For this review, take the finished solid that the model builds, in its own axes (mm). A direction names the side the tool comes from. Round coordinates to 2 decimals unless told otherwise and drop trailing zeros. Write each loop counter-clockwise with the first axis right and the second up, starting at its lowest first coordinate (ties: lowest second). Pieces come first, ordered by that corner, then holes. Notation, with made-up numbers: (-24, -26) -> (-12, -26) arc R20 ccw to (-12, -8) -> close; hole circle Ø5 at (-39.75, 74.25). An arc over 180 degrees is marked (long way). Write each question's results on one line, items separated by ' | '. Start each with the question number.
Item 1: To check wall thickness, follow line 1 along X through (y, z) = (107.5, 0) (3 decimals); line 2 along Y through (x, z) = (-3.5, -6); line 3 along X through (y, z) = (208, 4.75). State the ranges of each line that lie inside material, in increasing order.
Item 2: Add section B-B (y = 187). State the section outline as (x, z) points (3 decimals), plus the area to 3 significant figures.
Item 3: The part is to be moulded in two halves that separate along Z. For faces 1 (the cylindrical face through (3.86, 150.27, 5.04)), 2 (the cylindrical face through (1.93, 154.6, 2.52)), 3 (the flat face through (7, 304.8, 0)), say which applies: +Z half, -Z half, draft (parallel to the pull), parting line (faces both ways), or undercut.
Item 4: Add section A-A (x = 0). State the section outline as (y, z) points (3 decimals), plus the area to 3 significant figures.
Item 5: Clearance check with flat-ended pins moving along their axes: pin 1 (8 mm diameter, centred on x = 3, y = 146.5, fed in from -Z); pin 2 (2 mm diameter, centred on x = 5.5, y = 103.5, fed in from +Z); pin 3 (2 mm diameter, centred on x = 2, y = 65.5, fed in from +Z). State where each tip first meets the part, or that it passes through.
Item 6: Tool access review of faces 4 (the flat face through (7, 0, 0)), 5 (the flat face through (2, 309.8, -3)): name each direction out of +Z, -Z, +X, -X, +Y, -Y from which nothing blocks a thin tool from reaching the whole face with its end or side.
from build123d import *

# Parameters (mm, degrees)
SKETCH1_R            = 6.35
SKETCH1_R_2          = 3.175
BOSS_EXTRUDE1_DEPTH  = 304.8
SKETCH2_R            = 3.175
BOSS_EXTRUDE2_DEPTH  = 5
FILLET1_R            = 0.5
FILLET1_OF_MIRROR1_R = 0.5


with BuildPart() as part:
    # Sketch1 → Boss-Extrude1 (new body)
    with BuildSketch(Plane(origin=(0, 0, 0), x_dir=(1, 0, 0), z_dir=(0, 1, 0))):
        with Locations(Location((0, 0, 0), (0, 0, 90))):
            Circle(SKETCH1_R)
        with Locations(Location((0, 0, 0), (0, 0, 90))):
            Circle(SKETCH1_R_2, mode=Mode.SUBTRACT)
    extrude(amount=BOSS_EXTRUDE1_DEPTH)

    # Sketch2 → Boss-Extrude2 (add)
    with BuildSketch(Plane(origin=(0, 304.8, 0), x_dir=(1, 0, 0), z_dir=(0, 1, 0))):
        Polygon((-8.065583261, 0), (-4.03279163, -6.985), (4.03279163, -6.985), (8.065583261, 0), (4.03279163, 6.985), (-4.03279163, 6.985), align=None)
        with Locations(Location((0, 0, 0), (0, 0, 90))):
            Circle(SKETCH2_R, mode=Mode.SUBTRACT)
    boss_extrude2 = extrude(amount=BOSS_EXTRUDE2_DEPTH)

    # Fillet1
    fillet1_edges = [part.edges().sort_by_distance(p)[0] for p in [
        (-6.049187445, 309.8, -3.4925),
        (-6.049187445, 309.8, 3.4925),
        (0, 309.8, 6.985),
        (6.049187445, 309.8, 3.4925),
        (6.049187445, 309.8, -3.4925),
        (0, 309.8, -6.985),
        (-6.049187445, 304.8, -3.4925),
        (-4.03279163, 307.3, -6.985),
        (-6.049187445, 304.8, 3.4925),
        (-8.065583261, 307.3, 0),
        (0, 304.8, 6.985),
        (-4.03279163, 307.3, 6.985),
        (6.049187445, 304.8, 3.4925),
        (4.03279163, 307.3, 6.985),
        (6.049187445, 304.8, -3.4925),
        (8.065583261, 307.3, 0),
        (0, 304.8, -6.985),
        (4.03279163, 307.3, -6.985),
    ]]
    fillet(fillet1_edges, radius=FILLET1_R)

    # Mirror1: Boss-Extrude2 across plane
    add(boss_extrude2.mirror(Plane.ZX.offset(152.4)))

    # Fillet1 of Mirror1
    fillet1_of_mirror1_edges = [part.edges().sort_by_distance(p)[0] for p in [
        (-6.049187445, -5, -3.4925),
        (-6.049187445, -5, 3.4925),
        (0, -5, 6.985),
        (6.049187445, -5, 3.4925),
        (6.049187445, -5, -3.4925),
        (0, -5, -6.985),
        (-6.049187445, 0, -3.4925),
        (-4.03279163, -2.5, -6.985),
        (-6.049187445, 0, 3.4925),
        (-8.065583261, -2.5, 0),
        (0, 0, 6.985),
        (-4.03279163, -2.5, 6.985),
        (6.049187445, 0, 3.4925),
        (4.03279163, -2.5, 6.985),
        (6.049187445, 0, -3.4925),
        (8.065583261, -2.5, 0),
        (0, 0, -6.985),
        (4.03279163, -2.5, -6.985),
    ]]
    fillet(fillet1_of_mirror1_edges, radius=FILLET1_OF_MIRROR1_R)


solid = part.part
Responses:
1) line 1: x = -6.35 to -3.175, 3.175 to 6.35 | line 2: y = -5 to 0, 304.8 to 309.8 | line 3: x = -4.21 to 4.21
2) outline: circle Ø12.7 at (0, 0); hole circle Ø6.35 at (0, 0) | area: 95.0 mm^2
3) face 1: parting line | face 2: undercut | face 3: draft
4) outline: (-5, -6.485) arc R0.5 ccw to (-4.5, -6.985) -> (-0.5, -6.985) arc R0.5 ccw to (0, -6.485) -> (0, -6.35) -> (304.8, -6.35) -> (304.8, -6.485) arc R0.5 ccw to (305.3, -6.985) -> (309.3, -6.985) arc R0.5 ccw to (309.8, -6.485) -> (309.8, -3.175) -> (-5, -3.175) -> close; (-5, 3.175) -> (309.8, 3.175) -> (309.8, 6.485) arc R0.5 ccw to (309.3, 6.985) -> (305.3, 6.985) arc R0.5 ccw to (304.8, 6.485) -> (304.8, 6.35) -> (0, 6.35) -> (0, 6.485) arc R0.5 ccw to (-0.5, 6.985) -> (-4.5, 6.985) arc R0.5 ccw to (-5, 6.485) -> close | area: 2,010 mm^2
5) pin 1: stops at z = -6.35 | pin 2: stops at z = 4.48 | pin 3: stops at z = 6.27
6) face 4: none | face 5: +Z, -Z, +X, -X, +Y
